```python
from build123d import *

# Parameters (mm, degrees)
F1_DEPTH = 19.05


with BuildPart() as f1:
    # F0 (on Front) → F1 (new body)
    with BuildSketch(Plane.XZ):
        with BuildLine():
            Line((-609.6, -25.4), (609.6, -25.4))
            Line((609.6, -25.4), (609.6, 25.4))
            Line((609.6, 25.4), (545.833553, 25.4))
            ThreePointArc((545.833553, 25.4), (527.05, 9.525), (508.266447, 25.4))
            Line((508.266447, 25.4), (395.247839, 25.4))
            ThreePointArc((395.247839, 25.4), (376.464286, 9.525), (357.680732, 25.4))
            Line((357.680732, 25.4), (244.662125, 25.4))
            ThreePointArc((244.662125, 25.4), (225.878571, 9.525), (207.095018, 25.4))
            Line((207.095018, 25.4), (94.07641, 25.4))
            ThreePointArc((94.07641, 25.4), (75.292857, 9.525), (56.509304, 25.4))
            Line((56.509304, 25.4), (-56.509304, 25.4))
            ThreePointArc((-56.509304, 25.4), (-75.292857, 9.525), (-94.07641, 25.4))
            Line((-94.07641, 25.4), (-207.095018, 25.4))
            ThreePointArc((-207.095018, 25.4), (-225.878571, 9.525), (-244.662125, 25.4))
            Line((-244.662125, 25.4), (-357.680732, 25.4))
            ThreePointArc((-357.680732, 25.4), (-376.464286, 9.525), (-395.247839, 25.4))
            Line((-395.247839, 25.4), (-508.266447, 25.4))
            ThreePointArc((-508.266447, 25.4), (-527.05, 9.525), (-545.833553, 25.4))
            Line((-545.833553, 25.4), (-609.6, 25.4))
            Line((-609.6, 25.4), (-609.6, -25.4))
        make_face()
    extrude(amount=F1_DEPTH)


solid = f1.part
```
Check sheet for the modelled part. Datum: model origin and axes. Units: mm. Coordinates: 2 decimals unless noted, no trailing zeros. Order: outer loops, then holes, each group sorted by start corner. A loop starts at its lowest first (then second) coordinate and runs counter-clockwise, first axis right, second up. Notation, with made-up numbers: M 84,-7.5 L 112,-7.5 A26 ccw 112,6.5 Z; hole C 85,64 d7. An arc over 180 degrees is marked long. One line per question, with ' | ' between items. Start each with the question number.
Item 1: Sectioned sample at B-B on x = -81.5. Record the cut outline in (y, z).
Item 2: Material ranges on line 1 (Z direction, x = 380, y = -15.5); line 2 (Z direction, x = 517, y = -16.5), recorded low to high.
Item 3: Mould release check, pull along X, two halves, no side actions. Record for faces 1 (the flat face through (-609.6, -9, 0)), 2 (the flat face through (-9, 0, 0)), 3 (the cylindrical face through (226.25, -9.39, 9.53)): pulls with the +X half, pulls with the -X half, needs draft (parallel to the pull), parting line crosses it, or undercut.
Item 4: Sectioned sample at C-C on x = -527. Record the cut outline in (y, z), and give its area (3 significant figures).
Item 5: Gauge pin test, flat end, axial feed: P1, Ø4, axis at x = -221, y = -15, coming from the +Z side. Record the tip position at first contact, or that the pin passes through.
Item 6: Sectioned sample at A-A on y = -12.5. Record the cut outline in (x, z) (3 decimals), and give its area (3 significant figures).
Answer below:
1) outline: M -19.05,-25.4 L 0,-25.4 L 0,10.56 L -19.05,10.56 Z
2) line 1: z = -25.4 to 9.86 | line 2: z = -25.4 to 12.39
3) face 1: pulls with the -X half | face 2: needs draft | face 3: undercut
4) outline: M -19.05,-25.4 L 0,-25.4 L 0,9.53 L -19.05,9.53 Z | area: 665 mm^2
5) P1: stops at z = 10.81
6) outline: M -609.6,-25.4 L 609.6,-25.4 L 609.6,25.4 L 545.834,25.4 A19.05 cw 508.266,25.4 L 395.248,25.4 A19.05 cw 357.681,25.4 L 244.662,25.4 A19.05 cw 207.095,25.4 L 94.076,25.4 A19.05 cw 56.509,25.4 L -56.509,25.4 A19.05 cw -94.076,25.4 L -207.095,25.4 A19.05 cw -244.662,25.4 L -357.681,25.4 A19.05 cw -395.248,25.4 L -508.266,25.4 A19.05 cw -545.834,25.4 L -609.6,25.4 Z | area: 58,300 mm^2
